Could you check a few things on this model? Use its own coordinates, in mm. A direction names the side the tool comes from. Give positions to 0.01 mm unless a question says otherwise; leave off trailing zeros. Loops run counter-clockwise (first coordinate to the right, second up) from the corner with the lowest first, then second, coordinate; pieces in that order, holes last. Notation, with made-up numbers: (-21, 51.5) - (-10, 51.5) arc R16 ccw to (-10, 65.5) - close; hole circle Ø7 at (-11.5, 35.5). An arc over 180 degrees is marked (long way). Write each question's results on one line, items separated by ' | '. Start each with the question number.
(1) Suppose I cut it at C-C (y = -10). Please give me the cut outline in (x, z).
(2) Suppose I cut it at B-B (y = 27). Please give me the cut outline in (x, z).
(3) I need wall thicknesses on line 1 (X direction, y = 45, z = 6); line 2 (Y direction, x = -5, z = 7); line 3 (Y direction, x = 11, z = 1.25). Which ranges of each line are inside material? Lowest first, please.
(4) For pin 1 (0.6 mm diameter, centred on x = 13.5, y = 64, fed in from -Z); pin 2 (4 mm diameter, centred on x = 4, z = 6, fed in from -Y); pin 3 (12 mm diameter, centred on x = 21, y = -6, fed in from +Z), each with a flat end and sliding along its axis, tell me the tip position at first contact or that it passes through.
(5) Suppose I cut it at D-D (x = 14.5). Please give me the cut outline in (y, z).
(6) Suppose I cut it at A-A (x = -9.5). Please give me the cut outline in (y, z).
(7) If we mould it in two halves opening along Y, with no side actions, what happens to faces 1 (the face through (-0.1, -61.849, 9.5)), 2 (the face through (0, 63.5, 5)), 3 (the face through (-29.031, -61.972, 5.151))? For each: released by +Y, released by -Y, zero draft, split by the parting line, or undercut.
(8) On a 3-axis mill with a long thin cutter (end or side, diameter ignored), from which of +Z, -Z, +X, -X, +Y, -Y can I reach the whole of each face in a straight line? I mean faces 4 (the face through (15, 64.008, 5)), 5 (the face through (-27.81, 60.4, 6.3)). Say none if no direction works.
from build123d import *

# Parameters (mm, degrees)
F0_W      = 60.96
F0_H      = 127
F1_DEPTH  = 10.16
F2_W      = 58.674
F2_H      = 123.698
F3_DEPTH  = 7.62
F4_R      = 5.08
F5_R      = 5.08
F6_W      = 45.72
F6_H      = 5.842
F7_DEPTH  = 25.4
F8_R      = 1.016
F9_W      = 25.752777
F9_H      = 6.35
F10_DEPTH = 25.4
F11_W     = 13.145404
F11_H     = 3.033555
F12_DEPTH = 0.508
F13_R     = 0.762


with BuildPart() as f1:
    # F0 (on Top) → F1 (new body)
    with BuildSketch(Plane.XY):
        Rectangle(F0_W, F0_H)
    extrude(amount=F1_DEPTH)

    # F2 (on face) → F3 (cut)
    with BuildSketch(Plane.XY.offset(10.16)):
        Rectangle(F2_W, F2_H)
    extrude(amount=-F3_DEPTH, mode=Mode.SUBTRACT)

    # F4
    f4_edges = [f1.edges().sort_by_distance(p)[0] for p in [
        (-29.337, 61.849, 6.35),
    ]]
    fillet(f4_edges, radius=F4_R)

    # F5
    f5_edges = [f1.edges().sort_by_distance(p)[0] for p in [
        (29.337, 61.849, 6.35),
        (29.337, -61.849, 6.35),
        (-29.337, -61.849, 6.35),
        (30.48, 63.5, 5.08),
        (-30.48, 63.5, 5.08),
        (-30.48, -63.5, 5.08),
        (30.48, -63.5, 5.08),
    ]]
    fillet(f5_edges, radius=F5_R)

    # F6 (on face) → F7 (cut)
    with BuildSketch(Plane.XZ.offset(63.5)):
        with Locations((0, 5.956087)):
            Rectangle(F6_W, F6_H)
    extrude(amount=-F7_DEPTH, mode=Mode.SUBTRACT)

    # F8
    f8_edges = [f1.edges().sort_by_distance(p)[0] for p in [
        (-22.86, -62.6745, 8.877087),
        (22.86, -62.6745, 8.877087),
    ]]
    fillet(f8_edges, radius=F8_R)

    # F9 (on face) → F10 (cut)
    with BuildSketch(Plane(origin=(-30.48, 0, 0), x_dir=(0, -1, 0), z_dir=(-1, 0, 0))):
        with Locations((-31.762417, 6.265609)):
            Rectangle(F9_W, F9_H)
    extrude(amount=-F10_DEPTH, mode=Mode.SUBTRACT)

    # F11 (on face) → F12 (join)
    with BuildSketch(Plane(origin=(0, 63.5, 0), x_dir=(-1, 0, 0), z_dir=(0, 1, 0))):
        with Locations((-14.788578, 5.435118)):
            Rectangle(F11_W, F11_H)
    extrude(amount=F12_DEPTH)

    # F13
    f13_edges = [f1.edges().sort_by_distance(p)[0] for p in [
        (8.215876, 63.754, 3.918341),
        (8.215876, 63.754, 6.951896),
        (21.36128, 63.754, 3.918341),
        (21.36128, 63.754, 6.951896),
    ]]
    fillet(f13_edges, radius=F13_R)


solid = f1.part
Output values:
1) outline: (-30.48, 0) - (30.48, 0) - (30.48, 10.16) - (29.34, 10.16) - (29.34, 2.54) - (-29.34, 2.54) - (-29.34, 10.16) - (-30.48, 10.16) - close
2) outline: (-30.48, 0) - (30.48, 0) - (30.48, 10.16) - (29.34, 10.16) - (29.34, 2.54) - (-29.34, 2.54) - (-29.34, 3.09) - (-30.48, 3.09) - close; (-30.48, 9.44) - (-29.34, 9.44) - (-29.34, 10.16) - (-30.48, 10.16) - close
3) line 1: -30.48 to -29.34, 29.34 to 30.48 | line 2: 61.85 to 63.5 | line 3: -63.5 to 63.5
4) pin 1: z = 3.92 | pin 2: y = 61.85 | pin 3: z = 2.54
5) outline: (-63.5, 0) - (63.5, 0) - (63.5, 3.92) - (64.01, 3.92) - (64.01, 6.95) - (63.5, 6.95) - (63.5, 10.16) - (61.85, 10.16) - (61.85, 2.54) - (-61.85, 2.54) - (-61.85, 3.04) - (-63.5, 3.04) - close; (-63.5, 8.88) - (-61.85, 8.88) - (-61.85, 10.16) - (-63.5, 10.16) - close
6) outline: (-63.5, 0) - (63.5, 0) - (63.5, 10.16) - (61.85, 10.16) - (61.85, 2.54) - (-61.85, 2.54) - (-61.85, 3.04) - (-63.5, 3.04) - close; (-63.5, 8.88) - (-61.85, 8.88) - (-61.85, 10.16) - (-63.5, 10.16) - close
7) face 1: undercut | face 2: released by +Y | face 3: released by -Y
8) face 4: +Z, -Z, +X, -X, +Y | face 5: +Z
